```python
from build123d import *

# Parameters (mm, degrees)
AUFSATZ_LINEAR_AUSTRAGEN1_DEPTH    = 2
F_2_0_2_DURCHMESSER_BOHRUNG1_D     = 2
F_2_0_2_DURCHMESSER_BOHRUNG1_DEPTH = 2
F_2_0_2_DURCHMESSER_BOHRUNG1_TIP   = 0.600860619
SCHNITT_LINEAR_AUSTRAGEN1_DEPTH    = 0.7
FASE2_SIZE                         = 0.2


with BuildPart() as part:
    # Skizze1 → Aufsatz-Linear austragen1 (new body)
    with BuildSketch(Plane(origin=(0, 0, 0), x_dir=(0, 1, 0), z_dir=(0, 0, 1))):
        with BuildLine():
            Line((-3.5, 12.1), (3.5, 12.1))
            ThreePointArc((3.5, 12.1), (5.839273194, 12.328073296), (8.090437621, 13.0037028))
            ThreePointArc((8.090437621, 13.0037028), (11.348885271, 12.348885271), (12.0037028, 9.090437621))
            ThreePointArc((12.0037028, 9.090437621), (11.328073296, 6.839273194), (11.1, 4.5))
            Line((11.1, 4.5), (11.1, -4.5))
            ThreePointArc((11.1, -4.5), (8.874011537, -9.874011537), (3.5, -12.1))
            Line((3.5, -12.1), (-3.5, -12.1))
            ThreePointArc((-3.5, -12.1), (-5.839273194, -12.328073296), (-8.090437621, -13.0037028))
            ThreePointArc((-8.090437621, -13.0037028), (-11.348885271, -12.348885271), (-12.0037028, -9.090437621))
            ThreePointArc((-12.0037028, -9.090437621), (-11.328073296, -6.839273194), (-11.1, -4.5))
            Line((-11.1, -4.5), (-11.1, 4.5))
            ThreePointArc((-11.1, 4.5), (-8.874011537, 9.874011537), (-3.5, 12.1))
        make_face()
        with BuildLine():
            Line((-3.5, 8.3), (3.5, 8.3))
            ThreePointArc((3.5, 8.3), (6.187005769, 7.187005769), (7.3, 4.5))
            Line((7.3, 4.5), (7.3, -4.5))
            ThreePointArc((7.3, -4.5), (6.187005769, -7.187005769), (3.5, -8.3))
            Line((3.5, -8.3), (-3.5, -8.3))
            ThreePointArc((-3.5, -8.3), (-6.187005769, -7.187005769), (-7.3, -4.5))
            Line((-7.3, -4.5), (-7.3, 4.5))
            ThreePointArc((-7.3, 4.5), (-6.187005769, 7.187005769), (-3.5, 8.3))
        make_face(mode=Mode.SUBTRACT)
    extrude(amount=AUFSATZ_LINEAR_AUSTRAGEN1_DEPTH)

    # Ø2.0 (2) Durchmesser Bohrung1
    with Locations(Plane(origin=(0, 0, 2), x_dir=(0, -1, 0), z_dir=(0, 0, 1))):
        with Locations((-9.227564928, -10.227564928), (9.227564928, 10.227564928)):
            Hole(F_2_0_2_DURCHMESSER_BOHRUNG1_D / 2, depth=F_2_0_2_DURCHMESSER_BOHRUNG1_DEPTH)
            with Locations((0, 0, -(F_2_0_2_DURCHMESSER_BOHRUNG1_DEPTH + F_2_0_2_DURCHMESSER_BOHRUNG1_TIP / 2))):  # 118° drill point
                Cone(0, F_2_0_2_DURCHMESSER_BOHRUNG1_D / 2, F_2_0_2_DURCHMESSER_BOHRUNG1_TIP, mode=Mode.SUBTRACT)

    # Skizze5 → Schnitt-Linear austragen1 (cut)
    with BuildSketch(Plane(origin=(0, 0, 0), x_dir=(1, 0, 0), z_dir=(0, 0, -1))):
        with BuildLine():
            Line((4.5, -8.6), (-4.5, -8.6))
            ThreePointArc((-4.5, -8.6), (-8.106244584, -7.106244584), (-9.6, -3.5))
            Line((-9.6, -3.5), (-9.6, 3.5))
            ThreePointArc((-9.6, 3.5), (-8.106244584, 7.106244584), (-4.5, 8.6))
            Line((-4.5, 8.6), (4.5, 8.6))
            ThreePointArc((4.5, 8.6), (8.106244584, 7.106244584), (9.6, 3.5))
            Line((9.6, 3.5), (9.6, -3.5))
            ThreePointArc((9.6, -3.5), (8.106244584, -7.106244584), (4.5, -8.6))
        make_face()
    extrude(amount=-SCHNITT_LINEAR_AUSTRAGEN1_DEPTH, mode=Mode.SUBTRACT)

    # Fase2
    fase2_edges = [part.edges().sort_by_distance(p)[0] for p in [
        (0, 11.1, 2),
        (-8.3, 0, 2),
        (-7.187005769, 6.187005769, 2),
        (0, 7.3, 2),
        (0, 11.1, 0),
        (9.874011537, 8.874011537, 0),
        (12.1, 0, 0),
        (12.328073296, -5.839273194, 0),
        (12.348885271, -11.348885271, 0),
        (6.839273194, -11.328073296, 0),
        (0, -11.1, 0),
        (-9.874011537, -8.874011537, 0),
        (-12.1, 0, 0),
        (-12.328073296, 5.839273194, 0),
        (7.187005769, 6.187005769, 2),
        (-12.348885271, 11.348885271, 0),
        (-6.839273194, 11.328073296, 0),
        (8.3, 0, 2),
        (7.187005769, -6.187005769, 2),
        (0, -7.3, 2),
        (-6.839273194, 11.328073296, 2),
        (-12.348885271, 11.348885271, 2),
        (-12.328073296, 5.839273194, 2),
        (-12.1, 0, 2),
        (10.227564928, -10.227564928, 2),
        (10.227564928, -10.227564928, 0),
        (-9.874011537, -8.874011537, 2),
        (-7.187005769, -6.187005769, 2),
        (-10.227564928, 8.227564928, 2),
        (-10.227564928, 8.227564928, 0),
        (0, -11.1, 2),
        (6.839273194, -11.328073296, 2),
        (12.348885271, -11.348885271, 2),
        (12.328073296, -5.839273194, 2),
        (-8.106244584, 7.106244584, 0),
        (0, 8.6, 0),
        (8.106244584, 7.106244584, 0),
        (9.6, 0, 0),
        (8.106244584, -7.106244584, 0),
        (0, -8.6, 0),
        (-8.106244584, -7.106244584, 0),
        (12.1, 0, 2),
        (-9.6, 0, 0),
        (9.874011537, 8.874011537, 2),
    ]]
    chamfer(fase2_edges, length=FASE2_SIZE)


solid = part.part
```
Here's how the part is built. I have some questions about the finished solid (model axes, mm). A direction names the side the tool comes from. Give positions to 0.01 mm unless a question says otherwise; leave off trailing zeros. Order: outer loops, then holes, each group sorted by start corner. A loop starts at its lowest first (then second) coordinate and runs counter-clockwise, first axis right, second up. Notation, with made-up numbers: (15.5, 44.5) - (25.5, 44.5) arc R16 ccw to (25.5, 69.5) - close; hole circle Ø6 at (6.5, -7.75). An arc over 180 degrees is marked (long way). Answer as a JSON object with one key per item and string values. Group by question number.
Item 1: For P1, Ø1.2, axis at x = -1.5, z = 1.5, coming from the -Y side; P2, Ø1, axis at y = 8, z = 0.5, coming from the +X side; P3, Ø0.9, axis at y = 0.5, z = 1.5, coming from the -X side, each with a flat end and sliding along its axis, tell me the tip position at first contact or that it passes through.
Item 2: Please list where these lines run through material, in increasing order: probe 1 along X at (y, z) = (-1.75, 1.6); probe 2 along Y at (x, z) = (0.75, 1.6); probe 3 along X at (y, z) = (-6.25, 0.85).
Item 3: If we mould it in two halves opening along X, with no side actions, what happens to faces 1 (the flat face through (12.1, 0, 1)), 2 (the cylindrical face through (-12.322, 5.807, 0.989)), 3 (the cylindrical face through (-7.216, 6.157, 1.242))? For each: pulls with the +X half, pulls with the -X half, needs draft (parallel to the pull), parting line crosses it, or undercut.
Item 4: If we section it at B-B on y = 0.25: Please give me the cut outline in (x, z), and give its area (3 significant figures).
Item 5: If we section it at C-C on z = 1.15: Please give me the cut outline in (x, y), and give its area (3 significant figures).
Item 6: If we section it at A-A on x = 3.75: Please give me the cut outline in (y, z), and give its area (3 significant figures).
Item 7: Which directions (+Z, -Z, +X, -X, +Y, -Y) give clear straight access to the entire face, cutting with the end or side of a thin tool? Please do faces 4 (the flat face through (0, -11.1, 1)), 5 (the cylindrical face through (-7.157, -6.216, 1.242)), 6 (the flat face through (0, -8, 2)), 7 (the flat face through (0, -8, 0.7)).
Result set:
{
 "1": {"P1": "y = -11.1", "P2": "x = 10.96", "P3": "x = -12.1"},
 "2": {"probe 1": "-12.1 to -8.3, 8.3 to 12.1", "probe 2": "-11.1 to -7.3, 7.3 to 11.1", "probe 3": "-11.59 to -7.12, 7.12 to 12.42"},
 "3": {"face 1": "pulls with the +X half", "face 2": "pulls with the -X half", "face 3": "undercut"},
 "4": {"outline": "(-12.1, 0.2) - (-11.9, 0) - (-9.8, 0) - (-9.6, 0.2) - (-9.6, 0.7) - (-8.3, 0.7) - (-8.3, 1.8) - (-8.5, 2) - (-11.9, 2) - (-12.1, 1.8) - close; (8.3, 0.7) - (9.6, 0.7) - (9.6, 0.2) - (9.8, 0) - (11.9, 0) - (12.1, 0.2) - (12.1, 1.8) - (11.9, 2) - (8.5, 2) - (8.3, 1.8) - close", "area": "13.2 mm²"},
 "5": {"outline": "(-13, 8.09) arc R12.11 cw to (-12.1, 3.5) - (-12.1, -3.5) arc R7.6 ccw to (-4.5, -11.1) - (4.5, -11.1) arc R12.11 cw to (9.09, -12) arc R3 ccw to (13, -8.09) arc R12.11 cw to (12.1, -3.5) - (12.1, 3.5) arc R7.6 ccw to (4.5, 11.1) - (-4.5, 11.1) arc R12.11 cw to (-9.09, 12) arc R3 ccw to start; hole circle Ø2 at (-10.23, 9.23); hole (-8.3, -3.5) arc R3.8 ccw to (-4.5, -7.3) - (4.5, -7.3) arc R3.8 ccw to (8.3, -3.5) - (8.3, 3.5) arc R3.8 ccw to (4.5, 7.3) - (-4.5, 7.3) arc R3.8 ccw to (-8.3, 3.5) - close; hole circle Ø2 at (10.23, -9.23)", "area": "294 mm²"},
 "6": {"outline": "(-11.1, 0.2) - (-10.9, 0) - (-8.8, 0) - (-8.6, 0.2) - (-8.6, 0.7) - (-7.3, 0.7) - (-7.3, 1.8) - (-7.5, 2) - (-10.9, 2) - (-11.1, 1.8) - close; (7.3, 0.7) - (8.6, 0.7) - (8.6, 0.2) - (8.8, 0) - (10.9, 0) - (11.1, 0.2) - (11.1, 1.8) - (10.9, 2) - (7.5, 2) - (7.3, 1.8) - close", "area": "13.2 mm²"},
 "7": {"face 4": "+Z, -Z, -X, -Y", "face 5": "+Z, -Z", "face 6": "+Z, +X, -X, +Y, -Y", "face 7": "-Z"}
}
